from build123d import *

# Parameters (mm, degrees)
SKETCH_1_W          = 80
SKETCH_1_H          = 80
EXTRUDE_1_DEPTH     = 7.5
FILLET_1_R          = 4
SKETCH_2_W          = 6
SKETCH_2_H          = 6
SKETCH_2_W_2        = 8
SKETCH_2_H_2        = 4
CUT_EXTRUDE_1_DEPTH = 8


with BuildPart() as part:
    # 草图1 → 凸台-拉伸1 (new, symmetric)
    with BuildSketch(Plane(origin=(0, 0, 0), x_dir=(1, 0, 0), z_dir=(0, 1, 0))):
        Rectangle(SKETCH_1_W, SKETCH_1_H)
    extrude(amount=EXTRUDE_1_DEPTH, both=True)

    # 圆角1
    fillet_1_edges = [part.edges().sort_by_distance(p)[0] for p in [
        (-40, 7.5, 0),
        (0, 7.5, 40),
        (40, 7.5, 0),
        (0, 7.5, -40),
    ]]
    fillet(fillet_1_edges, radius=FILLET_1_R)

    # 草图2 → 切除-拉伸1 (cut)
    with BuildSketch(Plane.XY.offset(40)):
        with Locations((-35, -2.5)):
            Rectangle(SKETCH_2_W, SKETCH_2_H)
        with Locations((-21, -3.5)):
            Rectangle(SKETCH_2_W_2, SKETCH_2_H_2)
        with Locations((21, -3.5)):
            Rectangle(SKETCH_2_W_2, SKETCH_2_H_2)
        with Locations((35, -2.5)):
            Rectangle(SKETCH_2_W, SKETCH_2_H)
    extrude(amount=-CUT_EXTRUDE_1_DEPTH, mode=Mode.SUBTRACT)


solid = part.part
Input: part model. Units: mm. Frame: model coordinates. A direction names the side the tool comes from. Give positions to 0.01 mm unless a question says otherwise; leave off trailing zeros. Loops run counter-clockwise (first coordinate to the right, second up) from the corner with the lowest first, then second, coordinate; pieces in that order, holes last. Notation, with made-up numbers: M 46.5,26 L 95.5,26 A7 cw 95.5,33 Z; hole C -10.75,-26 d7. An arc over 180 degrees is marked long. Use one line per item in the form item = value.
1. Reachability of faces 1 (the face through (-38.859, 6.297, -0.56)), 2 (the face through (-25, -4, 36)) from +Z, -Z, +X, -X, +Y, -Y: full face, straight path, thin tool, end or side. Return the list, or none.
Numbers:
face_1 = +Z, -Z, -X, +Y
face_2 = +Z
2. First-contact query: pin 1 (4 mm diameter, centred on y = 4, z = -11.5, fed in from +X); pin 2 (1.8 mm diameter, centred on x = 36.5, y = -2.5, fed in from +Z). Flat tips, straight axial feed; report the tip coordinate or a pass-through.
Numbers:
pin_1 = 40
pin_2 = 32
3. Section query A-A, the plane y = -2.5. Return the cut outline in (x, z).
Numbers:
outline = M -40,-40 L 40,-40 L 40,40 L 38,40 L 38,32 L 32,32 L 32,40 L 25,40 L 25,32 L 17,32 L 17,40 L -17,40 L -17,32 L -25,32 L -25,40 L -32,40 L -32,32 L -38,32 L -38,40 L -40,40 Z
4. Pull-direction query (X, two-part tool) for faces 3 (the face through (-40, -2, 1)), 4 (the face through (-35, 0.5, 36)), 5 (the face through (40, -2, 1)), 6 (the face through (-1, 7.5, -1)); classes: released by +X, released by -X, zero draft, split by the parting line, or undercut.
Numbers:
face_3 = released by -X
face_4 = undercut
face_5 = released by +X
face_6 = zero draft
5. Line query: L1, parallel to Z at x = 33, y = -1.5. Output: solid intervals per line, ascending.
Numbers:
L1 = -40 to 32
